Drawing for the job (mm, zero at the part's lowest x, y, z). A direction names the side the tool comes from. Give positions to 0.01 mm unless a question says otherwise; leave off trailing zeros. Order: outer loops, then holes, each group sorted by start corner. A loop starts at its lowest first (then second) coordinate and runs counter-clockwise, first axis right, second up. Notation, with made-up numbers: M -18.75,-12.5 L 37.25,-12.5 A25 cw 37.25,9.5 Z; hole C -14.75,47 d7. An arc over 180 degrees is marked long. One line per item, written item: value.
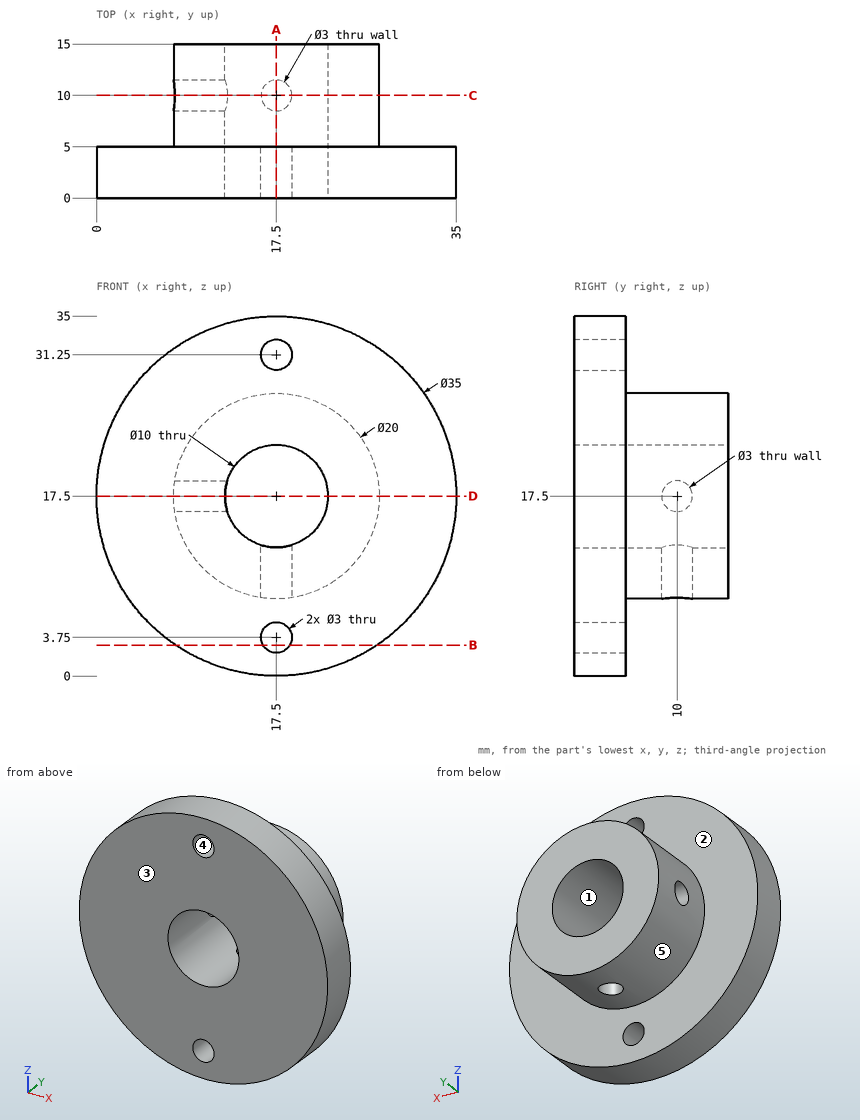
1) Mould opens along Z. For the marked faces 3, 4 and 5 say: released by +Z, released by -Z, zero draft, split by the parting line, or undercut.
Check values:
face 3: zero draft
face 4: undercut
face 5: split by the parting line
2) Saw through at D-D, the plane z = 17.5. Write the cut outline in (x, y).
Check values:
outline: M 0,0 L 12.5,0 L 12.5,8.5 L 7.5,8.5 L 7.5,5 L 0,5 Z; M 7.5,11.5 L 12.5,11.5 L 12.5,15 L 7.5,15 Z; M 22.5,0 L 35,0 L 35,5 L 27.5,5 L 27.5,15 L 22.5,15 Z
3) Saw through at B-B, the plane z = 3. Write the cut outline in (x, y), then the cut area to 3 significant figures.
Check values:
outline: M 7.7,0 L 16.2,0 L 16.2,5 L 7.7,5 Z; M 18.8,0 L 27.3,0 L 27.3,5 L 18.8,5 Z
area: 85.0 mm^2
4) Tool access for the marked faces 1 and 2: list every direction of +Z, -Z, +X, -X, +Y, -Y with a clear straight run to the whole face (end or side of a thin tool).
Check values:
face 1: +Y, -Y
face 2: +Y
5) Pin check, flat tips, straight feed: pin 1 (4 mm diameter, centred on y = 10, z = 17.5, fed in from +X); pin 2 (2 mm diameter, centred on x = 11, z = 3.5, fed in from +Y); pin 3 (3 mm diameter, centred on y = 2, z = 15.5, fed in from +X). Stop position of each tip, or through.
Check values:
pin 1: x = 27.5
pin 2: y = 5
pin 3: x = 34.99
6) Saw through at A-A, the plane x = 17.5. Write the cut outline in (y, z).
Check values:
outline: M 0,0 L 5,0 L 5,2.25 L 0,2.25 Z; M 0,5.25 L 5,5.25 L 5,7.5 L 8.5,7.5 L 8.5,12.5 L 0,12.5 Z; M 0,22.5 L 15,22.5 L 15,27.5 L 5,27.5 L 5,29.75 L 0,29.75 Z; M 0,32.75 L 5,32.75 L 5,35 L 0,35 Z; M 11.5,7.5 L 15,7.5 L 15,12.5 L 11.5,12.5 Z
7) Saw through at C-C, the plane y = 10. Write the cut outline in (x, z), then the cut area to 3 significant figures.
Check values:
outline: M 7.61,16 A10 ccw 16,7.61 L 16,12.73 A5 cw 12.73,16 Z; M 7.61,19 L 12.73,19 A5 cw long 19,12.73 L 19,7.61 A10 ccw long Z
area: 205 mm^2
8) Drill centre lines: probe 1 along Z at (x, y) = (17.5, 6.25); probe 2 along Y at (x, z) = (8.7, 17.5). Where is each one in solid material? Low to high. Write a range as from..to.
Check values:
probe 1: 7.5..12.5, 22.5..27.5
probe 2: 0..8.5, 11.5..15
